```python
from build123d import *

# Parameters (mm, degrees)
F0_R          = 7.5057
F0_R_2        = 2.9972
F1_DEPTH      = 10.9982
F2_R          = 1.4986
F3_DEPTH      = 7.5067
F3_DEPTH_BACK = 7.5067


with BuildPart() as f1:
    # F0 (on Front) → F1 (new body, symmetric)
    with BuildSketch(Plane.XZ):
        Circle(F0_R)
        Circle(F0_R_2, mode=Mode.SUBTRACT)
    extrude(amount=F1_DEPTH, both=True)

    # F2 (on Top) → F3 (cut, two sides)
    with BuildSketch(Plane.XY) as f3_sk:
        with Locations((0, 8.2042)):
            Circle(F2_R)
        with Locations((0, -8.2042)):
            Circle(F2_R)
    extrude(amount=F3_DEPTH, mode=Mode.SUBTRACT)
    extrude(f3_sk.sketch, amount=-F3_DEPTH_BACK, mode=Mode.SUBTRACT)


solid = f1.part
```
Here's how the part is built. I have some questions about the finished solid (model axes, mm). Coordinates: 2 decimals unless noted, no trailing zeros. Order: outer loops, then holes, each group sorted by start corner. A loop starts at its lowest first (then second) coordinate and runs counter-clockwise, first axis right, second up. Notation, with made-up numbers: (-2, 81) - (36, 81) arc R27 ccw to (36, 101) - close; hole circle Ø8 at (83.5, -2). An arc over 180 degrees is marked (long way). One line per question, with ' | ' between items. Start each with the question number.
1. Please list where these lines run through material, in increasing order: line 1 along Y through (x, z) = (0, -4.95); line 2 along Y through (x, z) = (-1.25, -6.25); line 3 along Z through (x, y) = (0, 2). Write a range as [from, to].
2. If we section it at C-C (y = -7.75): Write out the boundary of the cut face in (x, z).
3. I'm going to push flat-ended pins straight in: pin 1 Ø3.5 at (x, y) = (0, 8.2) entering from -Z; pin 2 Ø1 at (x, y) = (-4.5, -9) entering from -Z; pin 3 Ø1.5 at (x, y) = (-3.5, 5) entering from -Z; pin 4 Ø1.8 at (x, y) = (0, -8.2) entering from +Z. Where does each tip first touch, or does it pass through?
4. If we section it at B-B (x = 0): Write out the boundary of the cut face in (y, z), and give its area (3 significant figures).
5. If we section it at D-D (y = 0.5): Write out the boundary of the cut face in (x, z).
6. If we section it at A-A (z = 0): Write out the boundary of the cut face in (x, y), and give its area (3 significant figures).
7. If we mould it in two halves opening along X, with no side actions, what happens to faces 1 (the cylindrical face through (1.38, 0.15, -2.66)), 2 (the cylindrical face through (-1.627, -0.154, -7.327)), 3 (the flat face through (-0.1, -10.998, -3.2))? For each: released by +X, released by -X, zero draft, split by the parting line, or undercut.
Model answer:
1) line 1: y = [-11, -9.7], [-6.71, 6.71], [9.7, 11] | line 2: y = [-11, -9.03], [-7.38, 7.38], [9.03, 11] | line 3: z = [-7.51, -3], [3, 7.51]
2) outline: (-1.43, -7.37) - (-1.43, -2.64) arc R3 cw to (-1.43, 2.64) - (-1.43, 7.37) arc R7.51 ccw to start; (1.43, -7.37) arc R7.51 ccw to (1.43, 7.37) - (1.43, 2.64) arc R3 cw to (1.43, -2.64) - close
3) pin 1: stops at z = -7.51 | pin 2: stops at z = -6.35 | pin 3: stops at z = -6.98 | pin 4: passes through
4) outline: (-11, -7.51) - (-9.7, -7.51) - (-9.7, -3) - (-11, -3) - close; (-11, 3) - (-9.7, 3) - (-9.7, 7.51) - (-11, 7.51) - close; (-6.71, -7.51) - (6.71, -7.51) - (6.71, -3) - (-6.71, -3) - close; (-6.71, 3) - (6.71, 3) - (6.71, 7.51) - (-6.71, 7.51) - close; (9.7, -7.51) - (11, -7.51) - (11, -3) - (9.7, -3) - close; (9.7, 3) - (11, 3) - (11, 7.51) - (9.7, 7.51) - close | area: 144 mm²
5) outline: circle Ø15.01 at (0, 0); hole circle Ø5.99 at (0, 0)
6) outline: (-7.51, -11) - (-3, -11) - (-3, 11) - (-7.51, 11) - close; (3, -11) - (7.51, -11) - (7.51, 11) - (3, 11) - close | area: 198 mm²
7) face 1: undercut | face 2: split by the parting line | face 3: zero draft
